from build123d import *

# Parameters (mm, degrees)
SKETCH_1_R               = 50
EXTRUDE_1_DEPTH          = 20
SKETCH_4_R               = 12.5
CUT_EXTRUDE_1_DEPTH      = 40
EXTRUDE_2_REACH          = 115.578
EXTRUDE_2_END_RADIUS     = 50
SKETCH_5_W               = 13.960137626
SKETCH_5_H               = 22.640061842
SKETCH_6_W               = 13.960137626
SKETCH_6_H               = 22.640061842
EXTRUDE_3_DEPTH          = 100
EXTRUDE_4_DEPTH          = 80
EXTRUDE_4_DEPTH_BACK     = 20
SKETCH_7_R               = 7.782320826
SKETCH_13_R              = 79.451687304
CUT_EXTRUDE_2_DEPTH      = 16
SKETCH_14_R              = 50
EXTRUDE_5_DEPTH          = 16
SKETCH_17_W              = 12.089731424
SKETCH_17_H              = 31.60601215
EXTRUDE_6_DEPTH          = 50
CUT_EXTRUDE_3_DEPTH      = 15.831035086
CUT_EXTRUDE_4_REACH      = 292.221
CUT_EXTRUDE_4_END_RADIUS = 79.451687304
SKETCH_25_W              = 7.503169627
SKETCH_25_H              = 20.882263368
CUT_EXTRUDE_5_DEPTH      = 2
SKETCH_27_W              = 13.960137626
SKETCH_27_H              = 22.640061842
EXTRUDE_7_DEPTH          = 40


with BuildPart() as part:
    # Sketch 1 → Extrude 1 (new, symmetric)
    with BuildSketch(Plane.XY):
        Circle(SKETCH_1_R)
    extrude(amount=EXTRUDE_1_DEPTH, both=True)

    # Sketch 4 → Cut-Extrude 1 (cut)
    with BuildSketch(Plane.XY.offset(20)):
        with Locations((-25.673554091, -0.852792881)):
            Circle(SKETCH_4_R)
    extrude(amount=-CUT_EXTRUDE_1_DEPTH, mode=Mode.SUBTRACT)

    # Extrude 2: up to this cylinder (the profile starts outside it)
    extrude_2_end = Plane(origin=(0, 0, 0), z_dir=(0, 0, -1)) * Cylinder(EXTRUDE_2_END_RADIUS, 332.156, mode=Mode.PRIVATE)
    # Sketch 5 → Extrude 2 (add, up to the surface)
    with BuildSketch(Plane(origin=(50, 0, 0), x_dir=(0, 0, -1), z_dir=(1, 0, 0)), mode=Mode.PRIVATE) as extrude_2_sk1:
        Rectangle(SKETCH_5_W, SKETCH_5_H)
    extrude_2_tool1 = extrude(extrude_2_sk1.sketch, amount=-EXTRUDE_2_REACH, mode=Mode.PRIVATE) - extrude_2_end
    add(extrude_2_tool1.solids().sort_by_distance((50, 0, 0))[0])
    add(extrude_2_tool1.solids().sort_by_distance((50, 0, 0))[1])

    # Sketch 6 → Extrude 3 (add)
    with BuildSketch(Plane(origin=(50, 0, 0), x_dir=(0, 0, -1), z_dir=(1, 0, 0))):
        Rectangle(SKETCH_6_W, SKETCH_6_H)
    extrude(amount=EXTRUDE_3_DEPTH)

    # Sketch 7 → Extrude 4 (add, two sides: drawn at the far end of the back side and taken through both)
    with BuildSketch(Plane.XY.offset(6.980068813).offset(-EXTRUDE_4_DEPTH_BACK)):
        with Locations((134.496533675, 0)):
            Circle(SKETCH_7_R)
    extrude(amount=EXTRUDE_4_DEPTH + EXTRUDE_4_DEPTH_BACK)

    # Sketch 8 → Revolve 1 (revolve)
    with BuildSketch(Plane.XY.offset(86.980068813)):
        with BuildLine():
            Line((126.714212849, 0), (142.278854501, 0))
            ThreePointArc((142.278854501, 0), (134.496533675, -7.782320826), (126.714212849, 0))
        make_face()
    revolve(axis=Axis((126.714212849, 0, 86.980068813), (1, 0, 0)))

    # Sketch 10 → Revolve 2 (revolve)
    with BuildSketch(Plane(origin=(0, 0, 0), x_dir=(1, 0, 0), z_dir=(0, 1, 0))):
        Polygon((0, 20), (0, 44.4833931), (74.95212992, 44.4833931), (87.453253564, 17.178307248), (50, 17.178307248), (50, 20), align=None)
    revolve(axis=Axis((0, 0, -20), (0, 0, -1)))

    # Sketch 13 → Cut-Extrude 2 (cut)
    with BuildSketch(Plane.XY.offset(-17.178307248)):
        Circle(SKETCH_13_R)
    extrude(amount=-CUT_EXTRUDE_2_DEPTH, mode=Mode.SUBTRACT)


with BuildPart() as cut_extrude_2_piece_1:
    # of the separate pieces the step leaves, piece 1, a body of its own (cut_extrude_2_pieces)
    add(part.part.solids().sort_by_distance((50, 0, -17.178307248))[0])



with BuildPart() as cut_extrude_2_piece_2:
    # of the separate pieces the step leaves, piece 2, a body of its own (cut_extrude_2_pieces)
    add(part.part.solids().sort_by_distance((87.453253564, 0, -17.178307248))[0])


with BuildPart() as cut_extrude_2_piece_1_1:
    add(cut_extrude_2_piece_1.part)

    add(cut_extrude_2_piece_2.part)  # Extrude 5 merges Cut-Extrude 2 piece 2
    # Sketch 14 → Extrude 5 (add)
    with BuildSketch(Plane.XY.offset(-33.178307248)):
        Circle(SKETCH_14_R)
    extrude(amount=EXTRUDE_5_DEPTH)

    # Sketch 17 → Extrude 6 (add)
    with BuildSketch(Plane.ZY.offset(60)):
        with Locations((-23.392137874, 0)):
            Rectangle(SKETCH_17_W, SKETCH_17_H)
    extrude(amount=EXTRUDE_6_DEPTH)

    # Sketch 18 → Cut-Extrude 3 (cut)
    with BuildSketch(Plane.XY.offset(-17.347272162)):
        with BuildLine():
            Line((-77.864212669, 15.803006075), (-60, 15.803006075))
            Line((-60, 15.803006075), (-60, -15.803006075))
            Line((-60, -15.803006075), (-77.864212669, -15.803006075))
            ThreePointArc((-77.864212669, -15.803006075), (-79.451687304, 0), (-77.864212669, 15.803006075))
        make_face()
    extrude(amount=-CUT_EXTRUDE_3_DEPTH, mode=Mode.SUBTRACT)

    # Cut-Extrude 4: up to this cylinder (the profile starts outside it)
    cut_extrude_4_end = Plane(origin=(0, 0, -21.098857), z_dir=(0, 0, 1)) * Cylinder(CUT_EXTRUDE_4_END_RADIUS, 744.345374609, mode=Mode.PRIVATE)
    # Sketch 25 → Cut-Extrude 4 (cut, up to the surface)
    with BuildSketch(Plane.ZY.offset(110), mode=Mode.PRIVATE) as cut_extrude_4_sk1:
        with Locations((-21.098856975, 0)):
            Rectangle(SKETCH_25_W, SKETCH_25_H)
    cut_extrude_4_tool1 = extrude(cut_extrude_4_sk1.sketch, amount=-CUT_EXTRUDE_4_REACH, mode=Mode.PRIVATE) - cut_extrude_4_end
    add(cut_extrude_4_tool1.solids().sort_by_distance((-110, 0, -21.098857))[0], mode=Mode.SUBTRACT)

    # Sketch 26 → Cut-Extrude 5 (cut)
    with BuildSketch(Plane.XY.offset(-17.178307248)):
        with BuildLine():
            Line((-86.012727773, 15.807663329), (-77.863267306, 15.807663329))
            ThreePointArc((-77.863267306, 15.807663329), (-79.451687304, 0), (-77.863267306, -15.807663329))
            Line((-77.863267306, -15.807663329), (-86.012727773, -15.807663329))
            ThreePointArc((-86.012727773, -15.807663329), (-87.453253564, 0), (-86.012727773, 15.807663329))
        make_face()
    extrude(amount=-CUT_EXTRUDE_5_DEPTH, mode=Mode.SUBTRACT)

    # Sketch 27 → Extrude 7 (add)
    with BuildSketch(Plane(origin=(50, 0, 0), x_dir=(0, 0, -1), z_dir=(1, 0, 0))):
        Rectangle(SKETCH_27_W, SKETCH_27_H)
    extrude(amount=-EXTRUDE_7_DEPTH)


solid = cut_extrude_2_piece_1_1.part
CAD build for the part. Positions are in the model's coordinates, mm. A direction names the side the tool comes from. Give positions to 0.01 mm unless a question says otherwise; leave off trailing zeros. Write each loop counter-clockwise with the first axis right and the second up, starting at its lowest first coordinate (ties: lowest second). Pieces come first, ordered by that corner, then holes. Notation, with made-up numbers: M -25.75,-31.5 L 25.25,-31.5 A24 cw 25.25,1.5 Z; hole C 2.25,19.25 d5. An arc over 180 degrees is marked long. Put each result on its own line as item: value. Start each with the question number.
(1) Band-saw the part on A-A, the plane z = -22. Write the cut outline in (x, y), and give its area (3 significant figures).
(2) Band-saw the part on D-D, the plane z = 0.5. Write the cut outline in (x, y).
(3) Probe L1, parallel to Y at x = 0, z = -22.25; L2, parallel to Y at x = 26, z = -25; L3, parallel to X at y = 7, z = 8. List the from-to ranges inside material, lowest first.
(4) Band-saw the part on B-B, the plane x = -91. Write the cut outline in (y, z), and give its area (3 significant figures).
(5) Mould opens along Y. For faces 1 (the face through (-26, -1, -17.178)), 2 (the face through (-95, 0, -29.437)), 3 (the face through (72.237, -22.748, -42.775)) say: +Y half, -Y half, draft (parallel to the pull), parting line (faces both ways), or undercut.
(6) Which spindle directions (+Z, -Z, +X, -X, +Y, -Y) get a long thin tool onto all of the face, cutting with end or side? Do faces 4 (the face through (-95, 10.441, -21)), 5 (the face through (134, 0, -13.02)), 6 (the face through (126.72, 0.34, -10.04)), 7 (the face through (-35.59, -8.46, 1.67)), 8 (the face through (-98, -13, -17.347)). Say none if no direction does.
(7) Band-saw the part on C-C, the plane z = 17. Write the cut outline in (x, y).
(8) Flat gauge pins, fed straight in: pin 1 Ø10 at (x, z) = (73, 15) entering from -Y; pin 2 Ø12 at (x, z) = (44.5, 16.5) entering from +Y; pin 3 Ø18 at (x, y) = (93, 5) entering from -Z; pin 4 Ø15.5 at (x, z) = (100.5, 1.5) entering from +Y. Where does each tip first touch, or does it go through?
Response values:
1. outline: M -110,-15.8 L -83.77,-15.8 A85.25 ccw long -83.77,15.8 L -110,15.8 L -110,10.44 L -78.76,10.44 A79.45 cw long -78.76,-10.44 L -110,-10.44 Z; C 0,0 d100
1. area: 11,000 mm2
2. outline: M 48.7,-11.32 L 150,-11.32 L 150,11.32 L 48.7,11.32 A50 ccw long Z; hole C -25.67,-0.85 d25
3. L1: y = -85.13 to -79.45, -50 to 50, 79.45 to 85.13
3. L2: y = -79.74 to -75.08, -42.71 to 42.71, 75.08 to 79.74
3. L3: x = -49.51 to -35.4, -15.95 to 49.51, 131.1 to 137.9
4. outline: M -15.8,-29.44 L 15.8,-29.44 L 15.8,-17.35 L 10.44,-17.35 L 10.44,-24.85 L -10.44,-24.85 L -10.44,-17.35 L -15.8,-17.35 Z
4. area: 225 mm2
5. face 1: undercut
5. face 2: draft
5. face 3: parting line
6. face 4: +Z, -X
6. face 5: -Z, +X, +Y, -Y
6. face 6: -Z
6. face 7: +Z
6. face 8: +Z, -X, +Y, -Y
7. outline: C 0,0 d100; C 134.5,0 d15.56; hole C -25.67,-0.85 d25
8. pin 1: passes through
8. pin 2: stops at y = 31.9
8. pin 3: stops at z = -24.43
8. pin 4: stops at y = 11.32
